```python
from build123d import *

# Parameters (mm, degrees)
BOSS_EXTRUDE1_DEPTH = 2
SKETCH3_R           = 1.35
BOSS_EXTRUDE2_DEPTH = 3


with BuildPart() as part:
    # Sketch2 → Boss-Extrude1 (new body)
    with BuildSketch(Plane(origin=(0, 0, 0), x_dir=(1, 0, 0), z_dir=(0, 1, 0))):
        with BuildLine():
            Line((-36.5, -4), (36.5, -4))
            ThreePointArc((36.5, -4), (40.5, 0), (36.5, 4))
            Line((36.5, 4), (-36.5, 4))
            ThreePointArc((-36.5, 4), (-40.5, 0), (-36.5, -4))
        make_face()
    extrude(amount=BOSS_EXTRUDE1_DEPTH)

    # Sketch3 → Boss-Extrude2 (add)
    with BuildSketch(Plane(origin=(0, 2, 0), x_dir=(1, 0, 0), z_dir=(0, 1, 0))):
        with Locations(Location((-36.5, 0, 0), (0, 0, 270))):
            Circle(SKETCH3_R)
        with Locations(Location((36.5, 0, 0), (0, 0, 90))):
            Circle(SKETCH3_R)
    extrude(amount=BOSS_EXTRUDE2_DEPTH)


solid = part.part
```
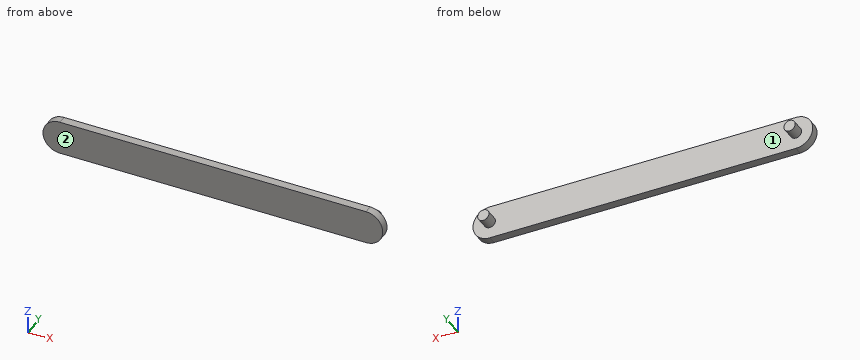
Input: part model. Units: mm. Frame: model coordinates. Face numbers are marked on the shaded views. Round coordinates to 2 decimals unless told otherwise and drop trailing zeros. Order: outer loops, then holes, each group sorted by start corner. A loop starts at its lowest first (then second) coordinate and runs counter-clockwise, first axis right, second up. Notation, with made-up numbers: (22, -10.75) - (65, -10.75) arc R38 cw to (65, 28.25) - close; hole circle Ø9 at (-13.75, 63.25). An arc over 180 degrees is marked (long way). One line per question, with ' | ' between items. Start each with the question number.
1) Cut plane A-A, the plane z = 0. Return the cut outline in (x, y).
2) Cut plane B-B, the plane x = -24. Return the cut outline in (y, z).
3) Contact query for flat-ended pins moving along their axis: P1, Ø4, axis at x = -15.5, z = -1.5, coming from the +Y side; P2, Ø1.5, axis at y = 3, z = -3, coming from the +X side; P3, Ø2, axis at y = 2.5, z = 1, coming from the -X side; P4, Ø2, axis at y = 3.5, z = -2, coming from the -X side. Output: stop coordinate, or through.
4) Pull-direction query (X, two-part tool) for the marked faces 1 and 2; classes: +X half, -X half, draft (parallel to the pull), parting line (faces both ways), or undercut.
5) Ray query, probe 1 along Y at (x, z) = (-3.5, 0); probe 2 along X at (y, z) = (2.75, 0.5); probe 3 along X at (y, z) = (3.75, 0.75). Return the intervals inside material, ascending.
Worked out:
1) outline: (-40.5, 0) - (40.5, 0) - (40.5, 2) - (37.85, 2) - (37.85, 5) - (35.15, 5) - (35.15, 2) - (-35.15, 2) - (-35.15, 5) - (-37.85, 5) - (-37.85, 2) - (-40.5, 2) - close
2) outline: (0, -4) - (2, -4) - (2, 4) - (0, 4) - close
3) P1: stops at y = 2 | P2: passes through | P3: stops at x = -40.5 | P4: stops at x = -37.41
4) face 1: undercut | face 2: draft
5) probe 1: y = 0 to 2 | probe 2: x = -37.75 to -35.25, 35.25 to 37.75 | probe 3: x = -37.62 to -35.38, 35.38 to 37.62
